```python
from build123d import *

# Parameters (mm, degrees)
SKETCH1_R           = 2
SKETCH1_W           = 12.7
SKETCH1_H           = 50.8
SKETCH1_R_2         = 12.095
SKETCH1_R_3         = 12.075
SKETCH1_R_4         = 1.143
BOSS_EXTRUDE1_DEPTH = 6.35
SKETCH5_R           = 2.75
CUT_EXTRUDE5_DEPTH  = 10


with BuildPart() as part:
    # Sketch1 → Boss-Extrude1 (new body)
    with BuildSketch(Plane(origin=(0, 0, 0), x_dir=(1, 0, 0), z_dir=(0, 1, 0))):
        with BuildLine():
            Line((-40.520093651, -53.074212293), (-34.358059191, -44.273915061))
            Line((-34.358059191, -44.273915061), (-29.852722948, -47.428585461))
            Line((-29.852722948, -47.428585461), (-36.014757408, -56.228882693))
            ThreePointArc((-36.014757408, -56.228882693), (-37.282182463, -61.682274385), (-34.419720881, -66.493943628))
            ThreePointArc((-34.419720881, -66.493943628), (-33.243515234, -66.777434912), (-32.240681933, -66.10056535))
            ThreePointArc((-32.240681933, -66.10056535), (-26.728650164, -59.250774979), (-19.793246149, -53.846860332))
            ThreePointArc((-19.793246149, -53.846860332), (-17.659799789, -51.192486841), (-17.721018114, -47.787557426))
            Line((-17.721018114, -47.787557426), (-22.618223277, -34.99005566))
            Line((-22.618223277, -34.99005566), (-17.481479686, -33.024383946))
            Line((-17.481479686, -33.024383946), (-12.584274523, -45.821885712))
            ThreePointArc((-12.584274523, -45.821885712), (-10.356790186, -48.397852623), (-6.996351286, -48.949887413))
            ThreePointArc((-6.996351286, -48.949887413), (0, -48.302004425), (6.996351286, -48.949887413))
            ThreePointArc((6.996351286, -48.949887413), (10.356790186, -48.397852623), (12.584274523, -45.821885712))
            Line((12.584274523, -45.821885712), (17.481479686, -33.024383946))
            Line((17.481479686, -33.024383946), (22.618223277, -34.99005566))
            Line((22.618223277, -34.99005566), (17.721018114, -47.787557426))
            ThreePointArc((17.721018114, -47.787557426), (17.659799789, -51.192486841), (19.793246149, -53.846860332))
            ThreePointArc((19.793246149, -53.846860332), (26.728650164, -59.250774979), (32.240681933, -66.10056535))
            ThreePointArc((32.240681933, -66.10056535), (33.243515234, -66.777434912), (34.419720881, -66.493943628))
            ThreePointArc((34.419720881, -66.493943628), (37.282182463, -61.682274385), (36.014757408, -56.228882693))
            Line((36.014757408, -56.228882693), (29.852722948, -47.428585461))
            Line((29.852722948, -47.428585461), (34.358059191, -44.273915061))
            Line((34.358059191, -44.273915061), (40.520093651, -53.074212293))
            ThreePointArc((40.520093651, -53.074212293), (45.927580176, -56.23617342), (51.848593315, -54.191543356))
            ThreePointArc((51.848593315, -54.191543356), (55.295899374, -50.669157408), (58.504414423, -46.927960674))
            ThreePointArc((58.504414423, -46.927960674), (60.030901261, -40.882046302), (56.458030011, -35.771485305))
            Line((56.458030011, -35.771485305), (56.349654942, -35.70891493))
            Line((56.349654942, -35.70891493), (47.078155187, -30.35601205))
            Line((47.078155187, -30.35601205), (49.828155187, -25.59287233))
            Line((49.828155187, -25.59287233), (59.099654942, -30.945775209))
            Line((59.099654942, -30.945775209), (59.208030011, -31.008345585))
            ThreePointArc((59.208030011, -31.008345585), (65.420341286, -31.547262353), (69.893013303, -27.202328787))
            ThreePointArc((69.893013303, -27.202328787), (73.860606951, 13.023468848), (56.374397975, 49.466425512))
            ThreePointArc((56.374397975, 49.466425512), (50.654117331, 52.01932544), (44.991624855, 49.340690033))
            Line((44.991624855, 49.340690033), (38.069871869, 41.091666046))
            Line((38.069871869, 41.091666046), (33.856627432, 44.626997899))
            Line((33.856627432, 44.626997899), (40.778380417, 52.876021886))
            ThreePointArc((40.778380417, 52.876021886), (42.433039833, 58.917628536), (38.925607882, 64.107698843))
            ThreePointArc((38.925607882, 64.107698843), (0, 75), (-38.925607882, 64.107698843))
            ThreePointArc((-38.925607882, 64.107698843), (-42.433039833, 58.917628536), (-40.778380417, 52.876021886))
            Line((-40.778380417, 52.876021886), (-33.856627432, 44.626997899))
            Line((-33.856627432, 44.626997899), (-38.069871869, 41.091666046))
            Line((-38.069871869, 41.091666046), (-44.991624855, 49.340690033))
            ThreePointArc((-44.991624855, 49.340690033), (-50.654117331, 52.01932544), (-56.374397975, 49.466425512))
            ThreePointArc((-56.374397975, 49.466425512), (-73.860606951, 13.023468848), (-69.893013303, -27.202328787))
            ThreePointArc((-69.893013303, -27.202328787), (-65.420341286, -31.547262353), (-59.208030011, -31.008345585))
            Line((-59.208030011, -31.008345585), (-59.099654942, -30.945775209))
            Line((-59.099654942, -30.945775209), (-49.828155187, -25.59287233))
            Line((-49.828155187, -25.59287233), (-47.078155187, -30.35601205))
            Line((-47.078155187, -30.35601205), (-56.349654942, -35.70891493))
            Line((-56.349654942, -35.70891493), (-56.458030011, -35.771485305))
            ThreePointArc((-56.458030011, -35.771485305), (-60.030901261, -40.882046302), (-58.504414423, -46.927960674))
            ThreePointArc((-58.504414423, -46.927960674), (-55.295899374, -50.669157408), (-51.848593315, -54.191543356))
            ThreePointArc((-51.848593315, -54.191543356), (-45.927580176, -56.23617342), (-40.520093651, -53.074212293))
        make_face()
        with Locations((-46.663733983, -40.081231883)):
            Circle(SKETCH1_R, mode=Mode.SUBTRACT)
        with Locations((-61.164123727, 0)):
            Rectangle(SKETCH1_W, SKETCH1_H, mode=Mode.SUBTRACT)
        with Locations((-32.995567884, -24.592872328)):
            Circle(SKETCH1_R_2, mode=Mode.SUBTRACT)
        with Locations((46.663733983, -40.081231883)):
            Circle(SKETCH1_R, mode=Mode.SUBTRACT)
        with Locations((0, -26.93833729)):
            Circle(SKETCH1_R_2, mode=Mode.SUBTRACT)
        with Locations((32.995567884, -24.592872328)):
            Circle(SKETCH1_R_2, mode=Mode.SUBTRACT)
        with Locations((61.164123727, 0)):
            Rectangle(SKETCH1_W, SKETCH1_H, mode=Mode.SUBTRACT)
        with Locations((-37.772386793, 25.4)):
            Circle(SKETCH1_R_3, mode=Mode.SUBTRACT)
        with Locations((-18.178952795, 24.310551096)):
            Circle(SKETCH1_R, mode=Mode.SUBTRACT)
        with Locations((-46.663733983, 40.081231883)):
            Circle(SKETCH1_R, mode=Mode.SUBTRACT)
        with Locations((-18.1962694, 47.045805056)):
            Circle(SKETCH1_R_2, mode=Mode.SUBTRACT)
        with Locations((-6.731, 64.107698843)):
            Circle(SKETCH1_R_4, mode=Mode.SUBTRACT)
        with Locations((0, 26.93833729)):
            Circle(SKETCH1_R_2, mode=Mode.SUBTRACT)
        with Locations((18.178952795, 24.310551096)):
            Circle(SKETCH1_R, mode=Mode.SUBTRACT)
        with Locations((37.772386793, 25.4)):
            Circle(SKETCH1_R_2, mode=Mode.SUBTRACT)
        with Locations((18.1962694, 47.045805056)):
            Circle(SKETCH1_R_2, mode=Mode.SUBTRACT)
        with Locations((0, 53.061187965)):
            Circle(SKETCH1_R, mode=Mode.SUBTRACT)
        with Locations((6.731, 64.107698843)):
            Circle(SKETCH1_R_4, mode=Mode.SUBTRACT)
        with Locations((46.663733983, 40.081231883)):
            Circle(SKETCH1_R, mode=Mode.SUBTRACT)
    extrude(amount=BOSS_EXTRUDE1_DEPTH)

    # Sketch5 → Cut-Extrude5 (cut)
    with BuildSketch(Plane(origin=(0, 6.35, 0), x_dir=(1, 0, 0), z_dir=(0, 1, 0))):
        with Locations((-48.453155187, -27.97444219)):
            Circle(SKETCH5_R)
        with Locations((-20.049851481, -34.007219803)):
            Circle(SKETCH5_R)
        with Locations((20.049851481, -34.007219803)):
            Circle(SKETCH5_R)
        with Locations((32.105391069, -45.851250261)):
            Circle(SKETCH5_R)
        with Locations((48.453155187, -27.97444219)):
            Circle(SKETCH5_R)
        with Locations((35.963249651, 42.859331973)):
            Circle(SKETCH5_R)
        with Locations((-35.963249651, 42.859331973)):
            Circle(SKETCH5_R)
    extrude(amount=-CUT_EXTRUDE5_DEPTH, mode=Mode.SUBTRACT)


solid = part.part
```
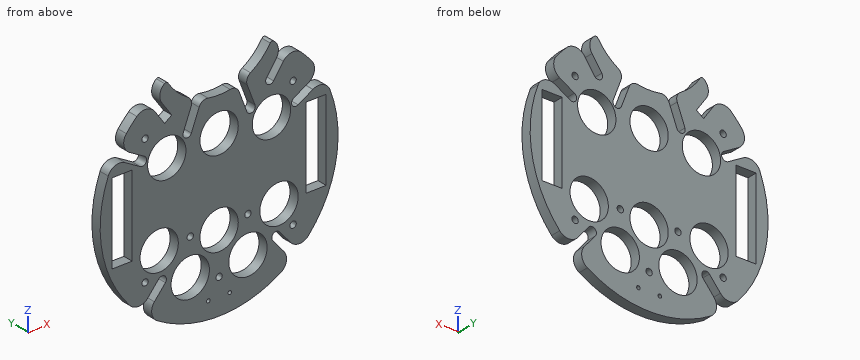
Geometry check sheet. Reference: the model listing, model coordinates, mm. Round coordinates to 2 decimals unless told otherwise and drop trailing zeros. Loops run counter-clockwise (first coordinate to the right, second up) from the corner with the lowest first, then second, coordinate; pieces in that order, holes last. Notation, with made-up numbers: M -4.5,-38.75 L 33.5,-38.75 A22 ccw 33.5,-6.75 Z; hole C 65.5,63.25 d7. An arc over 180 degrees is marked long. Return JSON: item names as keys, results as strings. Group by question number.
(1) Section check C-C, the plane z = -30.5. Enter the section's corners in (x, y).
(2) Section check D-D, the plane z = 0.5. Enter the section's corners in (x, y), and give its area (3 significant figures).
(3) Scan lines: line 1 along X through (y, z) = (1.5, -39.5); line 2 along X through (y, z) = (3.25, -9); line 3 along Z through (x, y) = (-40, 5.5). Record each from-to range of solid material in increasing order. Write a range as [from, to].
(4) Go/stop test with flat-tipped pins: pin 1 (1.5 mm diameter, centred on x = -30.5, y = 2, fed in from -Z); pin 2 (3 mm diameter, centred on x = -58, y = 3, fed in from -Z); pin 3 (1 mm diameter, centred on x = 0.5, y = 1, fed in from -Z). Record where each tip stops, or that it passes through.
(5) Section check B-B, the plane z = 18.5. Enter the section's corners in (x, y).
(6) Section check A-A, the plane x = 0. Enter the section's corners in (y, z).
Data:
{
 "1": {"outline": "M -68.52,0 L -48.72,0 L -48.72,6.35 L -68.52,6.35 Z; M -26.83,0 L -11.56,0 L -11.56,6.35 L -26.83,6.35 Z; M 11.56,0 L 26.81,0 L 26.81,6.35 L 11.56,6.35 Z; M 48.74,0 L 68.52,0 L 68.52,6.35 L 48.74,6.35 Z"},
 "2": {"outline": "M -75,0 L -67.51,0 L -67.51,6.35 L -75,6.35 Z; M -54.81,0 L 54.81,0 L 54.81,6.35 L -54.81,6.35 Z; M 67.51,0 L 75,0 L 75,6.35 L 67.51,6.35 Z", "area": "791 mm²"},
 "3": {"line 1": "[-63.76, -48.58], [-44.75, -27.65], [-8.74, 8.74], [27.65, 44.75], [48.58, 63.76]", "line 2": "[-74.46, -67.51], [-54.81, 54.81], [67.51, 74.46]", "line 3": "[-63.32, -51.95], [-43.39, -37.27], [-13.53, 14.73], [34.45, 52.33]"},
 "4": {"pin 1": "z = -68.85", "pin 2": "z = -49.32", "pin 3": "z = -75"},
 "5": {"outline": "M -72.68,0 L -67.51,0 L -67.51,6.35 L -72.68,6.35 Z; M -54.81,0 L -43.44,0 L -43.44,6.35 L -54.81,6.35 Z; M -22.55,0 L -8.67,0 L -8.67,6.35 L -22.55,6.35 Z; M 8.67,0 L 22.55,0 L 22.55,6.35 L 8.67,6.35 Z; M 43.44,0 L 54.81,0 L 54.81,6.35 L 43.44,6.35 Z; M 67.51,0 L 72.68,0 L 72.68,6.35 L 67.51,6.35 Z"},
 "6": {"outline": "M 0,-75 L 6.35,-75 L 6.35,-55.06 L 0,-55.06 Z; M 0,-51.06 L 6.35,-51.06 L 6.35,-39.03 L 0,-39.03 Z; M 0,-14.84 L 6.35,-14.84 L 6.35,14.84 L 0,14.84 Z; M 0,39.03 L 6.35,39.03 L 6.35,48.3 L 0,48.3 Z"}
}
